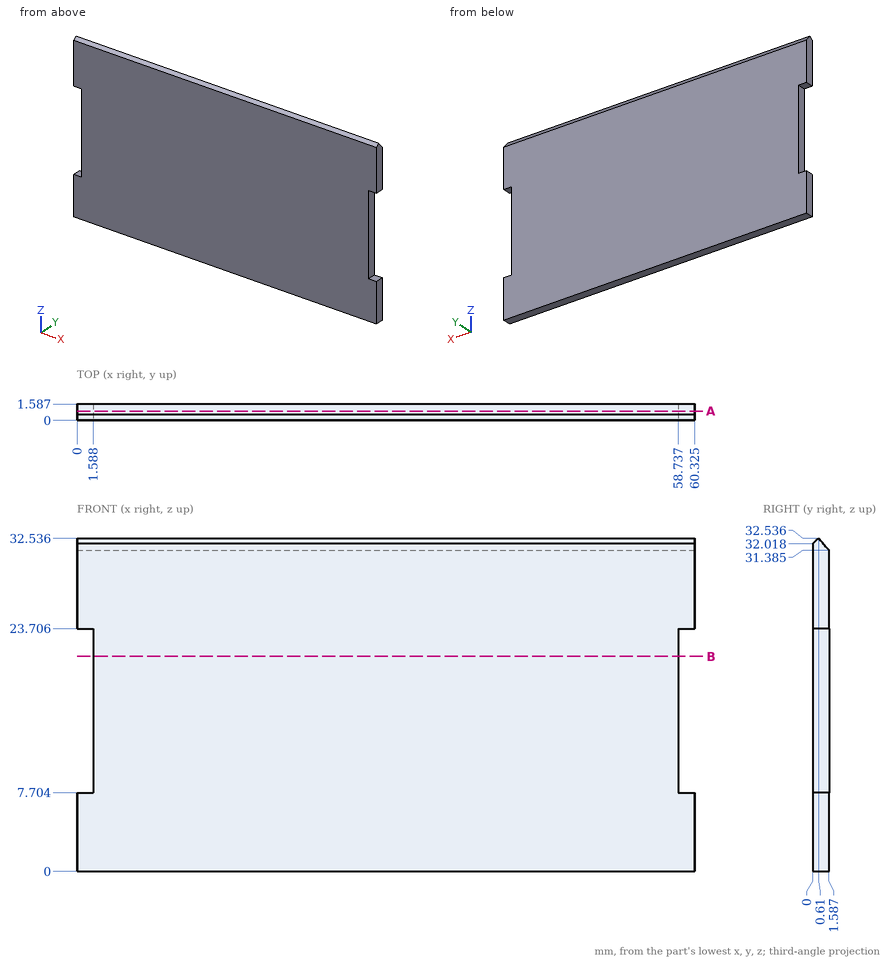
Could you check a few things on this drawing? It's one solid part, dimensions in mm from its lowest x, y, z. Give positions to 0.01 mm unless a question says otherwise; leave off trailing zeros. Write each loop counter-clockwise with the first axis right and the second up, starting at its lowest first coordinate (ties: lowest second). Pieces come first, ordered by that corner, then holes.
(1) Imagine slicing it at A-A, the plane y = 0.9. Write out the boundary of the cut face in (x, z) (1 decimal).
Output values:
outline: (0, 0) - (60.3, 0) - (60.3, 7.7) - (58.7, 7.7) - (58.7, 23.7) - (60.3, 23.7) - (60.3, 32.2) - (0, 32.2) - (0, 23.7) - (1.6, 23.7) - (1.6, 7.7) - (0, 7.7) - close
(2) Will these pins go through, and if not, where does the flat tip stop? pin 1 (3 mm diameter, centred on x = 47.5, z = 10, fed in from -Y); pin 2 (0.8 mm diameter, centred on y = 1, z = 19.5, fed in from +X); pin 3 (0.5 mm diameter, centred on y = 1, z = 12.5, fed in from -X).
Output values:
pin 1: stops at y = 0
pin 2: stops at x = 58.74
pin 3: stops at x = 1.59
(3) Imagine slicing it at B-B, the plane z = 21. Write out the boundary of the cut face in (x, y).
Output values:
outline: (1.59, 0) - (58.74, 0) - (58.74, 1.59) - (1.59, 1.59) - close
(4) If I drill on L1, parallel to Z at x = 22, y = 1.05 (1 decimal); L2, parallel to X at y = 1.25, z = 19; L3, parallel to Z at x = 12.5, y = 1.4 (1 decimal), over which ranges is the centre line in solid material (lowest first)?
Output values:
L1: z = 0 to 32
L2: x = 1.59 to 58.74
L3: z = 0 to 31.6
